Design review of the part built by this model. Coordinates are the model's own, in mm. A direction names the side the tool comes from. Coordinates: 2 decimals unless noted, no trailing zeros. Order: outer loops, then holes, each group sorted by start corner. A loop starts at its lowest first (then second) coordinate and runs counter-clockwise, first axis right, second up. Notation, with made-up numbers: (8.5, 71) -> (51.5, 71) arc R6 cw to (51.5, 80) -> close; hole circle Ø5 at (20, 17). An arc over 180 degrees is marked (long way). Use a Markdown table: item, result. Add a question column.
Q1. Add section A-A (x = 1.75). State the section outline as (y, z) points.
Q2. Wall thickness on probe 1 along Z at (x, y) = (4, 1.95); probe 2 along Y at (x, z) = (2, 1.25); probe 3 along Y at (x, z) = (6, 11.75): over which ranges is each line inside the solid? List them lowest first.
Q3. Machinability: for faces 5 (the face through (5.916, -7.285, -9.599)), 6 (the face through (8.43, -0.6, 0.18)), 7 (the face through (3.194, 1.521, 10.165)), which of the approach directions +Z, -Z, +X, -X, +Y, -Y give a long, thin tool a straight path to every point of the face, cutting with its end or side? Answer none if there is none.
Q4. Insertion check: pin 1 (1 mm diameter, centred on x = 3, z = 1, fed in from -Y); pin 2 (1.5 mm diameter, centred on y = -8.5, z = -4.5, fed in from -X). Each pin has a flat end and moves straight along its axis. Give the tip position at first contact, or say it passes through.
Q5. Add section B-B (y = -10.5). State the section outline as (x, z) points.
Q6. Add section D-D (x = 4). State the section outline as (y, z) points.
Q7. The part is to be moulded in two halves that separate along Y. For faces 1 (the face through (6, 3, 0)), 2 (the face through (3, 0, 0)), 3 (the face through (6, -10, -9.9)), 4 (the face through (8.4, -3.43, 0.18)), say which applies: pulls with the +Y half, pulls with the -Y half, needs draft (parallel to the pull), parting line crosses it, or undercut.
from build123d import *

# Parameters (mm, degrees)
BOSS_EXTRUDE1_DEPTH = 12.9
SKETCH2_W           = 3
SKETCH2_H           = 5
BOSS_EXTRUDE2_DEPTH = 12
SKETCH3_R           = 1.8
CUT_EXTRUDE1_DEPTH  = 5
FILLET1_R           = 2
FILLET2_R           = 1
SKETCH4_R           = 1.5
CUT_EXTRUDE2_DEPTH  = 3


with BuildPart() as part:
    # Sketch1 → Boss-Extrude1 (new, symmetric)
    with BuildSketch(Plane.XY):
        Polygon((0, 0), (9, 0), (9, -4), (0, -4), (0, -7), (12, -7), (12, 3), (0, 3), align=None)
    extrude(amount=BOSS_EXTRUDE1_DEPTH, both=True)

    # Sketch2 → Boss-Extrude2 (add, through all)
    with BuildSketch(Plane(origin=(12, 0, 0), x_dir=(0, 0, -1), z_dir=(1, 0, 0))):
        with Locations((-11.4, -9.5)):
            Rectangle(SKETCH2_W, SKETCH2_H)
        with Locations((11.4, -9.5)):
            Rectangle(SKETCH2_W, SKETCH2_H)
    extrude(amount=-BOSS_EXTRUDE2_DEPTH)

    # Sketch3 → Cut-Extrude1 (cut)
    with BuildSketch(Plane.XZ.offset(7)):
        with Locations((4, 0)):
            Circle(SKETCH3_R)
    extrude(amount=-CUT_EXTRUDE1_DEPTH, mode=Mode.SUBTRACT)

    # Fillet1
    fillet1_edges = [part.edges().sort_by_distance(p)[0] for p in [
        (9, -4, 0),
        (9, 0, 0),
    ]]
    fillet(fillet1_edges, radius=FILLET1_R - 0.0001)  # a hair under: the kernel refuses the full size

    # Fillet2
    fillet2_edges = [part.edges().sort_by_distance(p)[0] for p in [
        (6, -7, 9.9),
        (6, -7, -9.9),
    ]]
    fillet(fillet2_edges, radius=FILLET2_R)

    # Sketch4 → Cut-Extrude2 (cut)
    with BuildSketch(Plane(origin=(0, 3, 0), x_dir=(1, 0, 0), z_dir=(0, 1, 0))):
        with Locations(Location((4, 8.9, 0), (0, 0, 180))):
            Circle(SKETCH4_R)
        with Locations(Location((4, -8.9, 0), (0, 0, 180))):
            Circle(SKETCH4_R)
    extrude(amount=-CUT_EXTRUDE2_DEPTH, mode=Mode.SUBTRACT)


solid = part.part
Established:
| question | item | result |
|---|---|---|
| 1 | outline | (-12, -12.9) -> (-4, -12.9) -> (-4, 12.9) -> (-12, 12.9) -> (-12, 9.9) -> (-8, 9.9) arc R1 cw to (-7, 8.9) -> (-7, -8.9) arc R1 cw to (-8, -9.9) -> (-12, -9.9) -> close; (0, -12.9) -> (3, -12.9) -> (3, 12.9) -> (0, 12.9) -> close |
| 2 | probe 1 | -12.9 to -10.4, -7.4 to 7.4, 10.4 to 12.9 |
| 2 | probe 2 | -7 to -4, 0 to 3 |
| 2 | probe 3 | -12 to -4, 0 to 3 |
| 3 | face 5 | +X, -X, -Y |
| 3 | face 6 | +Z, -Z, -X |
| 3 | face 7 | +Y |
| 4 | pin 1 | y = -7 |
| 4 | pin 2 | through |
| 5 | outline | (0, -12.9) -> (12, -12.9) -> (12, -9.9) -> (0, -9.9) -> close; (0, 9.9) -> (12, 9.9) -> (12, 12.9) -> (0, 12.9) -> close |
| 6 | outline | (-12, -12.9) -> (-4, -12.9) -> (-4, -1.8) -> (-7, -1.8) -> (-7, -8.9) arc R1 cw to (-8, -9.9) -> (-12, -9.9) -> close; (-12, 9.9) -> (-8, 9.9) arc R1 cw to (-7, 8.9) -> (-7, 1.8) -> (-4, 1.8) -> (-4, 12.9) -> (-12, 12.9) -> close; (0, -12.9) -> (3, -12.9) -> (3, -10.4) -> (0, -10.4) -> close; (0, -7.4) -> (3, -7.4) -> (3, 7.4) -> (0, 7.4) -> close; (0, 10.4) -> (3, 10.4) -> (3, 12.9) -> (0, 12.9) -> close |
| 7 | face 1 | pulls with the +Y half |
| 7 | face 2 | undercut |
| 7 | face 3 | needs draft |
| 7 | face 4 | undercut |
